Could you check a few things on this model? Use its own coordinates, in mm. Face numbers are marked on the shaded views. A direction names the side the tool comes from. Round coordinates to 2 decimals unless told otherwise and drop trailing zeros. Loops run counter-clockwise (first coordinate to the right, second up) from the corner with the lowest first, then second, coordinate; pieces in that order, holes last.
from build123d import *

# Parameters (mm, degrees)
SKETCH_1_W          = 28
SKETCH_1_H          = 12
SKETCH_1_R          = 2.75
EXTRUDE_1_DEPTH     = 9.5
SKETCH_2_R          = 4.75
CUT_EXTRUDE_2_DEPTH = 5
SKETCH_3_R          = 4.5
CUT_EXTRUDE_3_DEPTH = 1281.252706776


with BuildPart() as part:
    # 草图1 → 拉伸1 (new body)
    with BuildSketch(Plane.XY):
        with Locations((1266.161217663, 1010.158991307)):
            Rectangle(SKETCH_1_W, SKETCH_1_H)
        with Locations((1274.161217663, 1010.158991307)):
            Circle(SKETCH_1_R, mode=Mode.SUBTRACT)
        with Locations((1258.161217663, 1010.158991307)):
            Circle(SKETCH_1_R, mode=Mode.SUBTRACT)
    extrude(amount=EXTRUDE_1_DEPTH)

    # 草图2 → 拉伸2 (cut)
    with BuildSketch(Plane(origin=(0, 0, 0), x_dir=(-1, 0, 0), z_dir=(0, 0, -1))):
        with Locations((-1258.161217663, 1010.158991307)):
            Circle(SKETCH_2_R)
        with Locations((-1274.161217663, 1010.158991307)):
            Circle(SKETCH_2_R)
    extrude(amount=-CUT_EXTRUDE_2_DEPTH, mode=Mode.SUBTRACT)

    # 草图3 → 拉伸3 (cut, through all)
    with BuildSketch(Plane(origin=(0, 1016.158991307, 0), x_dir=(1, 0, 0), z_dir=(0, 1, 0))):
        with Locations((1266.161217663, -10)):
            Circle(SKETCH_3_R)
    extrude(amount=-CUT_EXTRUDE_3_DEPTH, mode=Mode.SUBTRACT)


solid = part.part
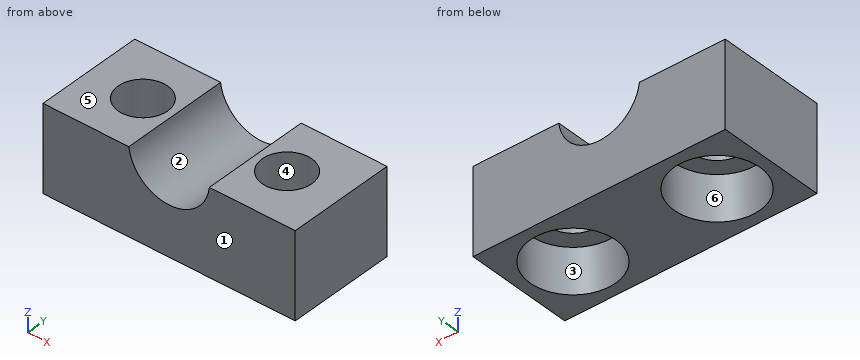
Item 1: For the marked faces 5 and 6, which set-ups out of +Z, -Z, +X, -X, +Y, -Y let a thin tool reach every point of the face, with its end or its side?
Results list:
face 5: +Z, +X, -X, +Y, -Y
face 6: -Z
Item 2: If we section it at C-C, the plane x = 1273.25: Please give me the cut outline in (y, z), then the cut area to 3 significant figures.
Results list:
outline: (1004.16, 0) - (1005.5, 0) - (1005.5, 5) - (1007.56, 5) - (1007.56, 9.5) - (1004.16, 9.5) - close; (1012.75, 5) - (1014.82, 5) - (1014.82, 0) - (1016.16, 0) - (1016.16, 9.5) - (1012.75, 9.5) - close
area: 44.0 mm2
Item 3: If I drill on line 1 along X through (y, z) = (1010.5, 8); line 2 along X through (y, z) = (1008.25, 2.75); line 3 along X through (y, z) = (1010, 6), over which ranges is the centre line in solid material (lowest first)?
Results list:
line 1: x = 1252.16 to 1255.43, 1260.89 to 1262.13, 1270.19 to 1271.43, 1276.89 to 1280.16
line 2: x = 1252.16 to 1253.81, 1262.51 to 1269.81, 1278.51 to 1280.16
line 3: x = 1252.16 to 1255.42, 1260.91 to 1264.1, 1268.22 to 1271.42, 1276.91 to 1280.16
Item 4: If we section it at D-D, the plane z = 6.25: Please give me the cut outline in (x, y).
Results list:
outline: (1252.16, 1004.16) - (1263.67, 1004.16) - (1263.67, 1016.16) - (1252.16, 1016.16) - close; (1268.65, 1004.16) - (1280.16, 1004.16) - (1280.16, 1016.16) - (1268.65, 1016.16) - close; hole circle Ø5.5 at (1258.16, 1010.16); hole circle Ø5.5 at (1274.16, 1010.16)
Item 5: We'd pull the mould along Y, two halves only. Please class the marked faces 1, 2, 3 and 4: released by +Y, released by -Y, zero draft, split by the parting line, or undercut.
Results list:
face 1: released by -Y
face 2: zero draft
face 3: undercut
face 4: undercut
Item 6: If we section it at B-B, the plane y = 1008.25: Please give me the cut outline in (x, z).
Results list:
outline: (1252.16, 0) - (1253.81, 0) - (1253.81, 5) - (1256.18, 5) - (1256.18, 9.5) - (1252.16, 9.5) - close; (1260.14, 5) - (1262.51, 5) - (1262.51, 0) - (1269.81, 0) - (1269.81, 5) - (1272.18, 5) - (1272.18, 9.5) - (1270.63, 9.5) arc R4.5 cw to (1261.69, 9.5) - (1260.14, 9.5) - close; (1276.14, 5) - (1278.51, 5) - (1278.51, 0) - (1280.16, 0) - (1280.16, 9.5) - (1276.14, 9.5) - close
Item 7: If we section it at A-A, the plane z = 8.5: Please give me the cut outline in (x, y).
Results list:
outline: (1252.16, 1004.16) - (1261.92, 1004.16) - (1261.92, 1016.16) - (1252.16, 1016.16) - close; (1270.4, 1004.16) - (1280.16, 1004.16) - (1280.16, 1016.16) - (1270.4, 1016.16) - close; hole circle Ø5.5 at (1258.16, 1010.16); hole circle Ø5.5 at (1274.16, 1010.16)
